from build123d import *

# Parameters (mm, degrees)
F0_R     = 1.6
F0_W     = 12.72
F0_H     = 12.72
F1_DEPTH = 6
F2_R     = 35
F3_R     = 20


with BuildPart() as f1:
    # F0 (on Top) → F1 (new body)
    with BuildSketch(Plane.XY):
        Polygon((25.6, 116.940437), (-14.9, 66.1), (-14.9, -14.9), (66.1, -14.9), (66.1, 66.1), align=None)
        with Locations((25.6, -7.45)):
            Circle(F0_R, mode=Mode.SUBTRACT)
        Polygon((0, 14.996133), (0, 36.203867), (14.996133, 51.2), (36.203867, 51.2), (51.2, 36.203867), (51.2, 14.996133), (36.203867, 0), (14.996133, 0), align=None, mode=Mode.SUBTRACT)
        with Locations((9.1, 66.1)):
            Circle(F0_R, mode=Mode.SUBTRACT)
        with Locations((42.1, 66.1)):
            Circle(F0_R, mode=Mode.SUBTRACT)
        with Locations((25.6, 88.46)):
            Rectangle(F0_W, F0_H, mode=Mode.SUBTRACT)
    extrude(amount=F1_DEPTH)

    # F2
    f2_edges = [f1.edges().sort_by_distance(p)[0] for p in [
        (66.1, -14.9, 3),
        (-14.9, -14.9, 3),
        (-14.9, 66.1, 3),
        (66.1, 66.1, 3),
    ]]
    fillet(f2_edges, radius=F2_R)

    # F3
    f3_edges = [f1.edges().sort_by_distance(p)[0] for p in [
        (25.6, 116.940437, 3),
    ]]
    fillet(f3_edges, radius=F3_R)


solid = f1.part
Build history of the part. All positions in model axes, mm. A direction names the side the tool comes from. Round coordinates to 2 decimals unless told otherwise and drop trailing zeros. Write each loop counter-clockwise with the first axis right and the second up, starting at its lowest first coordinate (ties: lowest second). Pieces come first, ordered by that corner, then holes. Notation, with made-up numbers: M 12,37.5 L 42,37.5 A15 cw 42,66.5 Z; hole C 6.25,83 d10. An arc over 180 degrees is marked long. Answer in a Markdown table with one row per item.
1. Saw through at B-B (y = 45.5). List the corners of the cut face in (x, z).
Geometry check:
| item | result |
|---|---|
| outline | M -14.9,0 L 9.3,0 L 9.3,6 L -14.9,6 Z; M 41.9,0 L 66.1,0 L 66.1,6 L 41.9,6 Z |
2. Saw through at C-C (z = 3). List the corners of the cut face in (x, y).
Geometry check:
| item | result |
|---|---|
| outline | M -14.9,20.1 A35 ccw 20.1,-14.9 L 31.1,-14.9 A35 ccw 66.1,20.1 L 66.1,53.86 A35 ccw 58.48,75.67 L 41.24,97.3 A20 ccw 9.96,97.3 L -7.28,75.67 A35 ccw -14.9,53.86 Z; hole M 0,15 L 15,0 L 36.2,0 L 51.2,15 L 51.2,36.2 L 36.2,51.2 L 15,51.2 L 0,36.2 Z; hole C 9.1,66.1 d3.2; hole M 19.24,82.1 L 31.96,82.1 L 31.96,94.82 L 19.24,94.82 Z; hole C 25.6,-7.45 d3.2; hole C 42.1,66.1 d3.2 |
3. Saw through at D-D (y = 66.1). List the corners of the cut face in (x, z).
Geometry check:
| item | result |
|---|---|
| outline | M -12.69,0 L 7.5,0 L 7.5,6 L -12.69,6 Z; M 10.7,0 L 40.5,0 L 40.5,6 L 10.7,6 Z; M 43.7,0 L 63.89,0 L 63.89,6 L 43.7,6 Z |
4. Which spindle directions (+Z, -Z, +X, -X, +Y, -Y) get a long thin tool onto all of the face, cutting with end or side? Do faces 1 (the face through (26, -14.9, 3)), 2 (the face through (0, 25, 3)). Say none if no direction does.
Geometry check:
| item | result |
|---|---|
| face 1 | +Z, -Z, +X, -X, -Y |
| face 2 | +Z, -Z |
5. Probe L1, parallel to Y at x = 9.1, z = 1.9; L2, parallel to X at y = 66.1, z = 3.2; L3, parallel to X at y = 21, z = 3.05. List the from-to ranges inside material, lowest first. Write a range as [from, to].
Geometry check:
| item | result |
|---|---|
| L1 | [-13.13, 5.9], [45.3, 64.5], [67.7, 96.23] |
| L2 | [-12.69, 7.5], [10.7, 40.5], [43.7, 63.89] |
| L3 | [-14.9, 0], [51.2, 66.1] |
6. Mould opens along X. For faces 3 (the face through (1.46, 86.64, 2.96)), 4 (the face through (64.084, 65.57, 3.042)), 5 (the face through (26, 82.1, 3)) say: +X half, -X half, draft (parallel to the pull), parting line (faces both ways), or undercut.
Geometry check:
| item | result |
|---|---|
| face 3 | -X half |
| face 4 | +X half |
| face 5 | undercut |
7. Flat gauge pins, fed straight in: P1, Ø2, axis at x = 45.5, z = 5, coming from the -Y side; P2, Ø3, axis at y = 86, z = 2, coming from the -X side; P3, Ø2, axis at x = -3.5, z = 4.5, coming from the +Y side. Where does each tip first touch, or does it go through?
Geometry check:
| item | result |
|---|---|
| P1 | y = -12.23 |
| P2 | x = -0.24 |
| P3 | y = 81.67 |
8. Saw through at A-A (x = 25.6). List the corners of the cut face in (y, z), and give its area (3 significant figures).
Geometry check:
| item | result |
|---|---|
| outline | M -14.9,0 L -9.05,0 L -9.05,6 L -14.9,6 Z; M -5.85,0 L 0,0 L 0,6 L -5.85,6 Z; M 51.2,0 L 82.1,0 L 82.1,6 L 51.2,6 Z; M 94.82,0 L 104.84,0 L 104.84,6 L 94.82,6 Z |
| area | 316 mm2 |
